Read the model definition and answer for the solid it produces. Units are mm, in the model's axes. Round coordinates to 2 decimals unless told otherwise and drop trailing zeros. Write each loop counter-clockwise with the first axis right and the second up, starting at its lowest first coordinate (ties: lowest second). Pieces come first, ordered by that corner, then holes. Notation, with made-up numbers: (1.5, 61) - (21.5, 61) arc R22 cw to (21.5, 76) - close; hole circle Ø7 at (-29.75, 62). An arc over 180 degrees is marked (long way). One line per item, written item: value. Start each with the question number.
(1) A cutting plane is placed at C-C, the plane y = 67.5. Determine the outline of the cut face in (x, z) (3 decimals), plus the area to 3 significant figures.
(2) A cutting plane is placed at A-A, the plane z = 0.95. State how many separate pieces and enclosed holes the cut face has, plus the area to 3 significant figures.
(3) Flat-ended cylindrical pins translate along their axes: pin 1 Ø3.5 at (x, y) = (139.7, 7.94) entering from -Z; pin 2 Ø4 at (x, y) = (107.95, 158.75) entering from -Z; pin 3 Ø1 at (y, z) = (150.5, 1) entering from +X; pin 4 Ø1.6 at (x, z) = (116.5, 1.5) entering from -Y. Find the tip coordinate at first contact, or state that the pin passes through.
(4) A cutting plane is placed at B-B, the plane x = 122. Determine the outline of the cut face in (y, z) (3 decimals).
(5) Find the intervals of material crossed by L1, parallel to X at y = 158.75, z = 2.25; L2, parallel to Y at x = 107.95, z = 1.5; L3, parallel to Y at x = 139.7, z = 0.95, in increasing order.
Autodesk Inventor part; units mm, degrees
ref_plane "YZ Plane" through (0, 0, 0) normal (1, 0, 0) x (0, 1, 0)
ref_plane "XZ Plane" through (0, 0, 0) normal (0, 1, 0) x (-1, 0, 0)
ref_plane "XY Plane" through (0, 0, 0) normal (0, 0, 1) x (1, 0, 0)
sketch "Sketch1" plane through (0, 0, 0) normal (0, 0, 1) x (1, 0, 0)
  line L0 (0, 0) -> (279.4, 0)
  line L1 (0, 0) -> (0, 165.1)
  line L2 (0, 165.1) -> (209.55, 165.1)
  line L3 (209.55, 165.1) -> (209.55, 114.3)
  line L4 (209.55, 114.3) -> (279.4, 0)
  circle A0 centre (9.525, 7.9375) radius 1.905
  circle A1 centre (98.425, 7.9375) radius 1.905
  line L5 (111.125, 0) -> (111.125, 25.4)
  line L6 (111.125, 25.4) -> (130.175, 25.4)
  line L7 (130.175, 25.4) -> (130.175, 0)
  circle A2 centre (12.7, 158.75) radius 1.5875
  circle A3 centre (107.95, 158.75) radius 1.5875
  circle A4 centre (203.2, 158.75) radius 1.5875
  circle A5 centre (12.7, 120.65) radius 1.5875
  circle A6 centre (107.95, 120.65) radius 1.5875
  circle A7 centre (203.2, 120.65) radius 1.5875
  circle A8 centre (139.7, 7.9375) radius 1.905
  circle A9 centre (257.175, 7.9375) radius 1.905
  line L8 (133.35, 0) -> (133.35, 15.875) construction
  line L9 (133.35, 0) -> (266.7, 0) construction
  line L10 (266.7, 15.875) -> (266.7, 0) construction
  line L11 (133.35, 15.875) -> (266.7, 15.875) construction
  dimension "d0" = 279.4
  dimension "d1" = 165.1
  dimension "d2" = 209.55
  dimension "d3" = 50.8
  dimension "d6" = 19.05
  dimension "d7" = 25.4
  dimension "d8" = 12.7
  dimension "d9" = 3.175
  dimension "d12" = 95.25
  dimension "d15" = 38.1
  dimension "d18" = 12.7
  dimension "d19" = 6.35
extrude "Extrusion1" add sketch "Sketch1" along normal blind 3.175 contours L1 L2 L3 L4 L0 L7 L6 L5
properties part number "Hopper Left Side Leg" material "Polycarbonate, Clear"
Here are the results:
1. outline: (0, 0) - (238.15, 0) - (238.15, 3.175) - (0, 3.175) - close
1. area: 756 mm²
2. separate pieces: 1
2. enclosed holes: 10
2. area: 38,000 mm²
3. pin 1: through
3. pin 2: z = 0
3. pin 3: x = 209.55
3. pin 4: y = 25.4
4. outline: (25.4, 0) - (165.1, 0) - (165.1, 3.175) - (25.4, 3.175) - close
5. L1: 0 to 11.11, 14.29 to 106.36, 109.54 to 201.61, 204.79 to 209.55
5. L2: 0 to 119.06, 122.24 to 157.16, 160.34 to 165.1
5. L3: 0 to 6.03, 9.84 to 165.1
